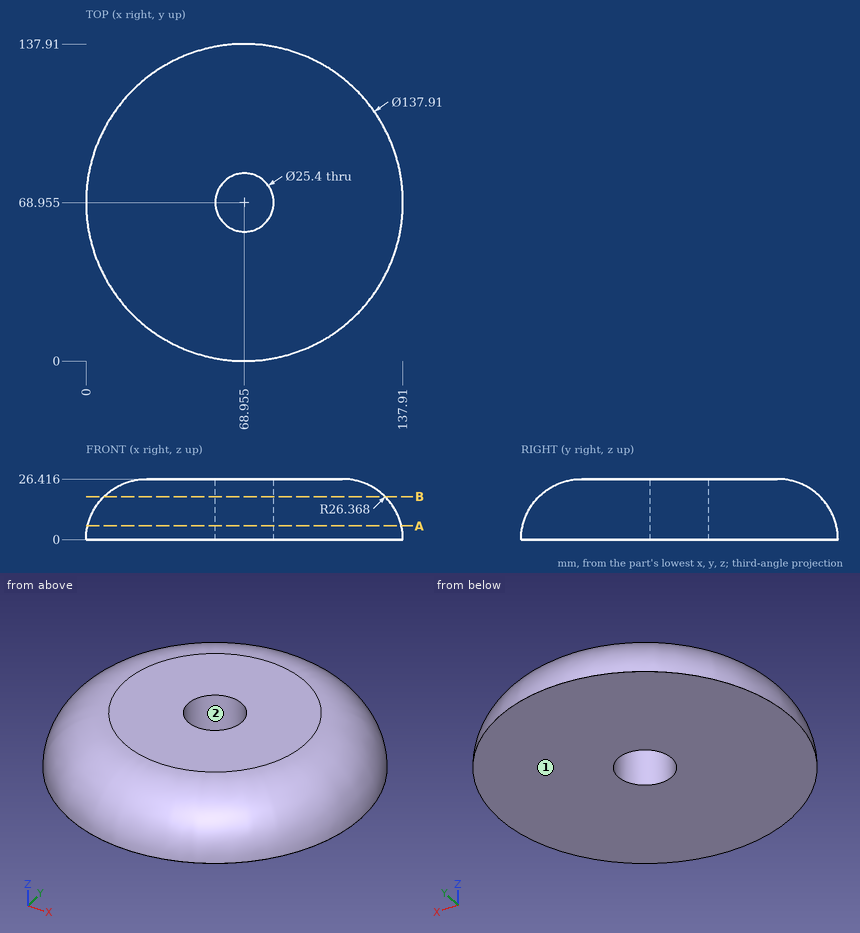
For this review, use the dimensioned drawing (mm, ordinates from the lowest corner) and the shaded views. Coordinates: 2 decimals unless noted, no trailing zeros. Write each loop counter-clockwise with the first axis right and the second up, starting at its lowest first coordinate (ties: lowest second). Pieces come first, ordered by that corner, then holes. Notation, with made-up numbers: (75.5, 7) -> (113.5, 7) arc R15 cw to (113.5, 17) -> close; hole circle Ø7 at (-17.5, 4.25). An arc over 180 degrees is marked (long way). Write each question's results on one line, items separated by ' | '. Start each with the question number.
(1) Take a section at A-A on z = 6. Write out the cut boundary in (x, y) (1 decimal), and give its area (3 significant figures).
(2) Take a section at B-B on z = 18.75. Write out the cut boundary in (x, y) (1 decimal).
(3) The part is to be moulded in two halves that separate along X. For the marked faces 1 and 2, say which applies: pulls with the +X half, pulls with the -X half, needs draft (parallel to the pull), parting line crosses it, or undercut.
(4) For line 1 along X through (y, z) = (60.5, 19.5); line 2 along Y through (x, z) = (68, 2.5); line 3 along X through (y, z) = (63.5, 11.75), list the stretches that pass through material, from the lowest coordinate up. Write a range as from..to.
(5) Clearance check with flat-ended pins moving along their axes: P1, Ø5, axis at x = 14.5, y = 108.5, coming from the +Z side; P2, Ø10, axis at x = 100.5, y = 32.5, coming from the +Z side; P3, Ø5, axis at x = 25.5, z = 23.5, coming from the -Y side. State where each tip first meets the part, or that it passes through.
Results found:
1) outline: circle Ø136.5 at (69, 69); hole circle Ø25.4 at (69, 69) | area: 14,100 mm2
2) outline: circle Ø122.3 at (69, 69); hole circle Ø25.4 at (69, 69)
3) face 1: needs draft | face 2: undercut
4) line 1: x = 9.16..59.48, 78.43..128.75 | line 2: y = 0.12..56.29, 81.62..137.79 | line 3: x = 2.96..57.49, 80.42..134.95
5) P1: stops at z = 14.26 | P2: stops at z = 26.41 | P3: stops at y = 28.95
